Can you work these out from the model? Positions are in its coordinate system, mm. Coordinates: 2 decimals unless noted, no trailing zeros. Order: outer loops, then holes, each group sorted by start corner. A loop starts at its lowest first (then second) coordinate and runs counter-clockwise, first axis right, second up. Notation, with made-up numbers: (47, 8) -> (83, 8) arc R32 cw to (83, 42) -> close; hole circle Ø8 at (59, 1). An arc over 180 degrees is marked (long way). Answer in a Markdown table with one row per item. Add a question column.
1. Will these pins go through, and if not, where does the flat tip stop? pin 1 (2 mm diameter, centred on x = -15, y = -1.5, fed in from -Z); pin 2 (2.5 mm diameter, centred on x = 10.5, z = -52, fed in from +Y); pin 3 (3 mm diameter, centred on y = 1, z = -50, fed in from +X); pin 4 (4 mm diameter, centred on x = -10.5, z = -58.5, fed in from -Y).
2. If I drill on line 1 along X through (y, z) = (0.75, -33.5); line 2 along X through (y, z) = (8.5, -83.5) (3 decimals); line 3 along Y through (x, z) = (18, -38.5), over which ranges is the centre line in solid material (lowest first)? Write a range as [from, to].
3. Imagine slicing it at A-A on y = 0. Write out the boundary of the cut face in (x, z).
from build123d import *

# Parameters (mm, degrees)
SKETCH1_R           = 2.5
BOSS_EXTRUDE1_DEPTH = 90
FILLET1_R           = 1.5


with BuildPart() as part:
    # Sketch1 → Boss-Extrude1 (new body)
    with BuildSketch(Plane.XY):
        Polygon((-1.499992211, 10), (2.38e-06, 10), (1.500001785, 10), (6.400001785, 10), (6.400001785, 9.479132912), (6.925001785, 9.479132912), (6.925001785, 8.2), (4.695347664, 8.2), (4.695347664, 6.8), (7.595347664, 3.9), (12.404655907, 3.9), (15.304655907, 6.94037733), (15.304655907, 8.199999348), (13.075001785, 8.199999348), (13.075001785, 9.565762703), (13.497472172, 9.573136951), (13.497472172, 9.999999348), (18.397472172, 9.999999348), (20.000001785, 10), (20.000001785, 8.503508491), (20.000001785, 8.500000005), (20.000001785, 3.600001911), (19.479137611, 3.600002038), (19.479137484, 3.075002038), (18.200004571, 3.075002348), (18.200005113, 5.30465647), (16.800005113, 5.30465681), (13.900004408, 2.404657514), (13.900003241, -2.404650729), (16.940379867, -5.304651467), (18.200002536, -5.304651773), (18.200003078, -3.074997652), (19.565766433, -3.074997983), (19.573140578, -3.497468372), (20.000002975, -3.497468476), (20.000001785, -8.397468476), (20.000001785, -10), (18.500003987, -10), (13.600003987, -9.99999881), (13.600004114, -9.479131722), (13.075004114, -9.479131595), (13.075004424, -8.199998683), (15.304655907, -8.199999224), (15.304655907, -6.8), (12.404655907, -3.9), (7.595347664, -3.9), (4.695347664, -6.94037733), (4.695347664, -8.2), (6.925001785, -8.2), (6.925001785, -9.565763355), (6.502531399, -9.573137603), (6.502531399, -10), (1.602531399, -10), (2.38e-06, -10), (-1.602527233, -10), (-6.502525798, -10), (-6.502525798, -9.573137078), (-6.92499762, -9.565763355), (-6.92499762, -8.2), (-4.695343498, -8.2), (-4.695343498, -6.94037733), (-7.595343498, -3.9), (-12.404651741, -3.9), (-15.304651741, -6.8), (-15.304651741, -8.2), (-13.07499762, -8.2), (-13.07499762, -9.479132912), (-13.600001017, -9.479132912), (-13.600001017, -10), (-18.49999954, -10), (-19.99999762, -10), (-19.99999762, -3.497471822), (-19.573134698, -3.497471822), (-19.565760974, -3.075), (-18.19999762, -3.075), (-18.19999762, -5.304654122), (-16.94037495, -5.304654122), (-13.89999762, -2.404654122), (-13.89999762, 2.404654122), (-16.79999762, 5.304654122), (-18.19999762, 5.304654122), (-18.19999762, 3.075), (-19.479130532, 3.075), (-19.479130532, 3.600003398), (-19.99999762, 3.600003398), (-19.99999762, 10), (-13.497469442, 10), (-13.497469442, 9.573137078), (-13.07499762, 9.565763355), (-13.07499762, 8.2), (-15.304651741, 8.2), (-15.304651741, 6.94037733), (-12.404651741, 3.9), (-7.595343498, 3.9), (-4.695343498, 6.8), (-4.695343498, 8.2), (-6.92499762, 8.2), (-6.92499762, 9.479132912), (-6.399994222, 9.479132912), (-6.399994222, 10), align=None)
        with Locations((-9.99999762, 0)):
            Circle(SKETCH1_R, mode=Mode.SUBTRACT)
        with Locations((9.99999762, 0)):
            Circle(SKETCH1_R, mode=Mode.SUBTRACT)
        Polygon((-3.059620289, 5.304654122), (-3.059620289, 8.2), (2.38e-06, 8.2), (3.059624455, 8.2), (3.059624455, 5.304654122), (6.100001785, 2.404654122), (6.100001785, -2.404654122), (3.200001785, -5.304654122), (3.200001785, -8.2), (2.38e-06, -8.2), (-3.19999762, -8.2), (-3.19999762, -5.304654122), (-6.09999762, -2.404654122), (-6.09999762, 2.404654122), align=None, mode=Mode.SUBTRACT)
    extrude(amount=-BOSS_EXTRUDE1_DEPTH)

    # Fillet1
    fillet1_edges = [part.edges().sort_by_distance(p)[0] for p in [
        (20.000001785, 10, -45),
        (20.000001785, -10, -45),
        (-19.99999762, -10, -45),
        (-19.99999762, 10, -45),
    ]]
    fillet(fillet1_edges, radius=FILLET1_R - 0.0001)  # a hair under: the kernel refuses the full size


solid = part.part
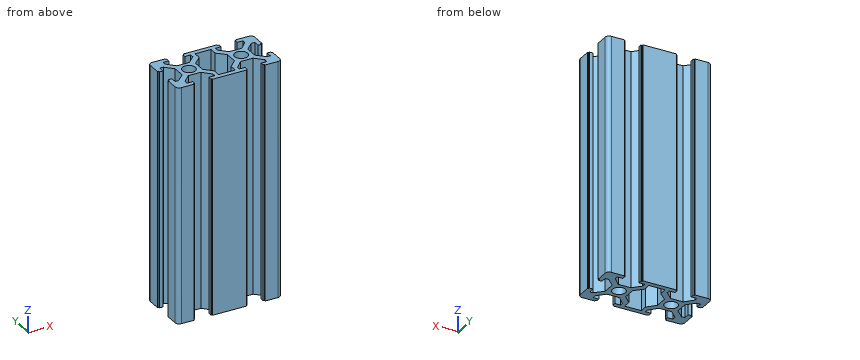
Answers follow:
| question | item | result |
|---|---|---|
| 1 | pin 1 | passes through |
| 1 | pin 2 | stops at y = 3.9 |
| 1 | pin 3 | stops at x = 14 |
| 1 | pin 4 | stops at y = -4 |
| 2 | line 1 | x = [-13.9, -12.38], [-7.62, -6.1], [6.1, 7.62], [12.38, 13.9] |
| 2 | line 2 | x = [-20, -13.075], [-6.925, 6.925], [13.075, 20] |
| 2 | line 3 | y = [-10, -5.3], [5.3, 10] |
| 3 | outline | (-13.9, -90) -> (-12.5, -90) -> (-12.5, 0) -> (-13.9, 0) -> close; (-7.5, -90) -> (-6.1, -90) -> (-6.1, 0) -> (-7.5, 0) -> close; (6.1, -90) -> (7.5, -90) -> (7.5, 0) -> (6.1, 0) -> close; (12.5, -90) -> (13.9, -90) -> (13.9, 0) -> (12.5, 0) -> close |
